Input: part model. Units: mm. Frame: model coordinates. A direction names the side the tool comes from. Coordinates: 2 decimals unless noted, no trailing zeros. Order: outer loops, then holes, each group sorted by start corner. A loop starts at its lowest first (then second) coordinate and runs counter-clockwise, first axis right, second up. Notation, with made-up numbers: (80, -32) -> (87, -32) arc R25 ccw to (87, -15) -> close; hole circle Ø4 at (51.5, 56.5). An arc over 180 degrees is marked (long way). One line per question, with ' | ' between items.
```python
from build123d import *

# Parameters (mm, degrees)
ESQUISSE1_R             = 7.5
BOSS_EXTRU_1_DEPTH      = 35
ESQUISSE2_R             = 4.875
ENL_V_MAT_EXTRU_1_DEPTH = 16
ESQUISSE3_R             = 4.05
ENL_V_MAT_EXTRU_2_DEPTH = 16
BOSS_EXTRU_3_START      = 9
BOSS_EXTRU_3_DEPTH      = 9


with BuildPart() as part:
    # Esquisse1 → Boss.-Extru.1 (new body)
    with BuildSketch(Plane(origin=(0, 0, 0), x_dir=(0, 1, 0), z_dir=(0, 0, 1))):
        with Locations(Location((0, 0, 0), (0, 0, 270))):
            Circle(ESQUISSE1_R)
    extrude(amount=BOSS_EXTRU_1_DEPTH)

    # Esquisse2 → Enlèv. mat.-Extru.1 (cut)
    with BuildSketch(Plane.XY.offset(35)):
        Circle(ESQUISSE2_R)
    extrude(amount=-ENL_V_MAT_EXTRU_1_DEPTH, mode=Mode.SUBTRACT)

    # Esquisse3 → Enlèv. mat.-Extru.2 (cut)
    with BuildSketch(Plane(origin=(0, 0, 0), x_dir=(1, 0, 0), z_dir=(0, 0, -1))):
        with Locations(Location((0, 0, 0), (0, 0, 180))):
            Circle(ESQUISSE3_R)
    extrude(amount=-ENL_V_MAT_EXTRU_2_DEPTH, mode=Mode.SUBTRACT)

    # Esquisse5 → Boss.-Extru.3 (add)
    with BuildSketch(Plane(origin=(0, 0, 16), x_dir=(1, 0, 0), z_dir=(0, 0, -1)).offset(BOSS_EXTRU_3_START)):
        with BuildLine():
            Line((-2.822041762, 2.904923458), (3.200496338, 2.481798378))
            ThreePointArc((3.200496338, 2.481798378), (0.283840932, 4.040041377), (-2.822041762, 2.904923458))
        make_face()
    extrude(amount=-BOSS_EXTRU_3_DEPTH)


solid = part.part
```
1. Ray query, line 1 (Y direction, x = 0, z = 5.75); line 2 (Z direction, x = 2.5, y = -0.75); line 3 (Y direction, x = 0, z = 8.75). Return the intervals inside material, ascending. Write a range as [from, to].
Recorded:
line 1: y = [-7.5, -4.05], [4.05, 7.5] | line 2: z = [16, 19] | line 3: y = [-7.5, -2.71], [4.05, 7.5]
2. Cut plane B-B, the plane y = 0. Return loops of the section in (x, z) (3 decimals), and give its area (3 significant figures).
Recorded:
outline: (-7.5, 0) -> (-4.05, 0) -> (-4.05, 16) -> (4.05, 16) -> (4.05, 0) -> (7.5, 0) -> (7.5, 35) -> (4.875, 35) -> (4.875, 19) -> (-4.875, 19) -> (-4.875, 35) -> (-7.5, 35) -> close | area: 239 mm^2
3. Access query for faces 1 (the face through (3, -3, 0)), 2 (the face through (0, 0, 19)), 3 (the face through (0, 1, 16)). Directions: +Z, -Z, +X, -X, +Y, -Y. A direction counts if a zero-diameter tool reaches every point of the face in a straight line with its end or side. Return the directions, or none.
Recorded:
face 1: -Z, +X, -X, +Y, -Y | face 2: +Z | face 3: -Z
4. Cut plane C-C, the plane x = 4.5. Return loops of the section in (y, z) (3 decimals), and give its area (3 significant figures).
Recorded:
outline: (-6, 0) -> (6, 0) -> (6, 35) -> (1.875, 35) -> (1.875, 19) -> (-1.875, 19) -> (-1.875, 35) -> (-6, 35) -> close | area: 360 mm^2
5. Cut plane D-D, the plane z = 31. Return loops of the section in (x, y) (3 decimals), and give its area (3 significant figures).
Recorded:
outline: circle Ø15 at (0, 0); hole circle Ø9.75 at (0, 0) | area: 102 mm^2
6. Pin query (flat end, axial travel): pin 1 Ø0.8 at (x, y) = (-0.5, -3.5) entering from -Z; pin 2 Ø2 at (x, y) = (-1.5, 3.5) entering from +Z; pin 3 Ø1 at (y, z) = (-5.5, 24.5) entering from -X. Return the tip coordinate at first contact, or that it passes through.
Recorded:
pin 1: stops at z = 7 | pin 2: stops at z = 19 | pin 3: stops at x = -5.59
7. Cut plane A-A, the plane z = 8.5. Return loops of the section in (x, y).
Recorded:
outline: circle Ø15 at (0, 0); hole (-2.82, -2.9) -> (3.2, -2.48) arc R4.05 ccw (long way) to start
8. Mould query, pull axis Y, two halves, no side actions, for faces 4 (the face through (-7.493, 0.33, 17.255)), 5 (the face through (2, -5, 35)), 6 (the face through (0.527, 4.016, 7.888)). Classes: released by +Y, released by -Y, zero draft, split by the parting line, or undercut.
Recorded:
face 4: split by the parting line | face 5: zero draft | face 6: undercut
